Part model, mm, in its own coordinate system. Give positions to 0.01 mm unless a question says otherwise; leave off trailing zeros. Order: outer loops, then holes, each group sorted by start corner. A loop starts at its lowest first (then second) coordinate and runs counter-clockwise, first axis right, second up.
1. Slice it at C-C on z = 1.5. Give the number of separate pieces and of enclosed holes in the cut face, and give its area (3 significant figures).
2. Slice it at D-D on y = 9.5. List the corners of the cut face in (x, z), and give its area (3 significant figures).
3. Slice it at A-A on x = 0. List the corners of the cut face in (y, z), and give its area (3 significant figures).
4. Slice it at B-B on y = 28.5. List the corners of the cut face in (x, z), and give its area (3 significant figures).
5. Mould opens along Y. For faces 1 (the cylindrical face through (-4.415, -31.136, 1.972)), 2 (the flat face through (7, 33.5, 2)), 3 (the flat face through (8.5, -3, 2)), 4 (the cylindrical face through (3.8, 11.1, 2)) say: +Y half, -Y half, draft (parallel to the pull), parting line (faces both ways), or undercut.
6. Probe line 1 (Y direction, x = -4.2, z = 1.7); line 2 (Y direction, x = -5.5, z = 2.8); line 3 (X direction, y = -17.5, z = 0.6). List the from-to ranges inside material, lowest first.
7. Drop flat-ended pins along their axis: pin 1 Ø5.5 at (x, y) = (-4.2, 9.5) entering from +Z; pin 2 Ø2.5 at (x, y) = (4.2, -29.5) entering from +Z. Give the stop position or say it passes through.
Autodesk Inventor part; units mm, degrees
ref_plane "YZ Plane" through (0, 0, 0) normal (1, 0, 0) x (0, 1, 0)
ref_plane "XZ Plane" through (0, 0, 0) normal (0, 1, 0) x (-1, 0, 0)
ref_plane "XY Plane" through (0, 0, 0) normal (0, 0, 1) x (1, 0, 0)
sketch "Skizze1" plane through (0, 0, 0) normal (0, 0, 1) x (1, 0, 0)
  line L0 (-8.5, -35) -> (8.5, -35)
  line L1 (8.5, -35) -> (8.5, 30.7574)
  line L2 (4.2574, 35) -> (-4.2574, 35)
  line L3 (-8.5, 30.7574) -> (-8.5, -35)
  line L4 (-12.1954, 0) -> (12.1954, 0)
  line L5 (0, -49.0422) -> (0, 49.2532)
  circle A0 centre (0, 28.5) radius 3.15
  circle A1 centre (-4.2, -29.5) radius 1.65
  circle A2 centre (4.2, -29.5) radius 1.65
  circle A3 centre (-4.2, -16.5) radius 1.65
  circle A4 centre (4.2, -16.5) radius 1.65
  circle A5 centre (-4.2, -3.5) radius 1.65
  circle A6 centre (4.2, -3.5) radius 1.65
  circle A7 centre (-4.2, 9.5) radius 1.65
  circle A8 centre (4.2, 9.5) radius 1.65
  line L6 (-6.3787, 34.1213) -> (-7.6213, 32.8787)
  line L7 (6.3787, 34.1213) -> (7.6213, 32.8787)
  arc A9 (8.5, 30.7574) -> (7.6213, 32.8787) centre (5.5, 30.7574) ccw
  arc A10 (6.3787, 34.1213) -> (4.2574, 35) centre (4.2574, 32) ccw
  arc A11 (-4.2574, 35) -> (-6.3787, 34.1213) centre (-4.2574, 32) ccw
  arc A12 (-7.6213, 32.8787) -> (-8.5, 30.7574) centre (-5.5, 30.7574) ccw
  point P0 (0, 0)
  point P1 (8.5, 35)
  point P2 (-8.5, 35)
  point P3 (-5.5, 35)
  point P4 (-8.5, 32)
  point P5 (5.5, 35)
  point P6 (8.5, 32)
  dimension "d0" = 17
  dimension "d1" = 70
  dimension "d2" = 6.3
  dimension "d3" = 6.5
  dimension "d4" = 3.3
  dimension "d5" = 3.3
  dimension "d6" = 3.3
  dimension "d7" = 3.3
  dimension "d8" = 3.3
  dimension "d9" = 3.3
  dimension "d10" = 3.3
  dimension "d11" = 3.3
  dimension "d12" = 4.3
  dimension "d13" = 8.4
  dimension "d14" = 5.5
  dimension "d15" = 13
  dimension "d16" = 13
  dimension "d17" = 13
  dimension "d18" = 3
  dimension "d19" = 3
  dimension "d20" = 3
  dimension "d21" = 3
  dimension "d24" = 3
extrude "Extrusion1" add sketch "Skizze1" along normal blind 4 contours L3 L4 L5 L0 | L5 L4 L1 L0 | L3 A12 L6 A11 L2 L5 A0 L4 | L5 A0 L2 A10 L7 A9 L1 L4
equation "\"d4\" = d5"
equation "\"d6\" = d5"
equation "\"d7\" = d5"
equation "\"d8\" = d5"
equation "\"d9\" = d5"
equation "\"d10\" = d5"
equation "\"d11\" = d5"
properties part number "Part2_new" material "Aluminium 6061"
Data:
1. separate pieces: 1
1. enclosed holes: 9
1. area: 1,080 mm2
2. outline: (-8.5, 0) - (-5.85, 0) - (-5.85, 4) - (-8.5, 4) - close; (-2.55, 0) - (2.55, 0) - (2.55, 4) - (-2.55, 4) - close; (5.85, 0) - (8.5, 0) - (8.5, 4) - (5.85, 4) - close
2. area: 41.6 mm2
3. outline: (-35, 0) - (25.35, 0) - (25.35, 4) - (-35, 4) - close; (31.65, 0) - (35, 0) - (35, 4) - (31.65, 4) - close
3. area: 255 mm2
4. outline: (-8.5, 0) - (-3.15, 0) - (-3.15, 4) - (-8.5, 4) - close; (3.15, 0) - (8.5, 0) - (8.5, 4) - (3.15, 4) - close
4. area: 42.8 mm2
5. face 1: undercut
5. face 2: +Y half
5. face 3: draft
5. face 4: undercut
6. line 1: y = -35 to -31.15, -27.85 to -18.15, -14.85 to -5.15, -1.85 to 7.85, 11.15 to 35
6. line 2: y = -35 to -30.52, -28.48 to -17.52, -15.48 to -4.52, -2.48 to 8.48, 10.52 to 34.73
6. line 3: x = -8.5 to -5.51, -2.89 to 2.89, 5.51 to 8.5
7. pin 1: stops at z = 4
7. pin 2: passes through
